from build123d import *

# Parameters (mm, degrees)
SKETCH_1_R          = 3
EXTRUDE_1_DEPTH     = 1
SKETCH_2_R          = 1.5
EXTRUDE_2_DEPTH     = 4
FILLET_1_R          = 0.4
CUT_EXTRUDE_1_DEPTH = 0.7
CHAMFER_1_SIZE      = 0.1
CHAMFER_2_SIZE      = 0.3


with BuildPart() as part:
    # 草图1 → 凸台-拉伸1 (new body)
    with BuildSketch(Plane.XY):
        Circle(SKETCH_1_R)
    extrude(amount=EXTRUDE_1_DEPTH)

    # 草图2 → 凸台-拉伸2 (add)
    with BuildSketch(Plane(origin=(0, 0, 0), x_dir=(-1, 0, 0), z_dir=(0, 0, -1))):
        Circle(SKETCH_2_R)
    extrude(amount=EXTRUDE_2_DEPTH)

    # 圆角1
    fillet_1_edges = [part.edges().sort_by_distance(p)[0] for p in [
        (-3, 0, 0),
        (-3, 0, 1),
    ]]
    fillet(fillet_1_edges, radius=FILLET_1_R)

    # 草图3 → 切除-拉伸1 (cut)
    with BuildSketch(Plane.XY.offset(1)):
        Polygon((0.343622422, -1.10238694), (1.126506305, -0.253607723), (0.782883884, 0.848779216), (-0.343622422, 1.10238694), (-1.126506305, 0.253607723), (-0.782883884, -0.848779216), align=None)
    extrude(amount=-CUT_EXTRUDE_1_DEPTH, mode=Mode.SUBTRACT)

    # 倒角1
    chamfer_1_edges = [part.edges().sort_by_distance(p)[0] for p in [
        (-0.219630731, -0.975583078, 0.3),
        (-0.954695095, -0.297585747, 0.3),
        (-0.735064364, 0.677997331, 0.3),
        (0.219630731, 0.975583078, 0.3),
        (0.954695095, 0.297585747, 0.3),
        (0.735064364, -0.677997331, 0.3),
        (-0.219630731, -0.975583078, 1),
        (0.735064364, -0.677997331, 1),
        (0.954695095, 0.297585747, 1),
        (0.219630731, 0.975583078, 1),
        (-0.735064364, 0.677997331, 1),
        (-0.954695095, -0.297585747, 1),
    ]]
    chamfer(chamfer_1_edges, length=CHAMFER_1_SIZE)

    # 倒角2
    chamfer_2_edges = [part.edges().sort_by_distance(p)[0] for p in [
        (1.5, 0, -4),
    ]]
    chamfer(chamfer_2_edges, length=CHAMFER_2_SIZE)


solid = part.part
Design review of the part built by this model. Coordinates are the model's own, in mm. A direction names the side the tool comes from. Give positions to 0.01 mm unless a question says otherwise; leave off trailing zeros. Order: outer loops, then holes, each group sorted by start corner. A loop starts at its lowest first (then second) coordinate and runs counter-clockwise, first axis right, second up. Notation, with made-up numbers: (30, 33) - (78, 33) arc R16 ccw to (78, 58) - close; hole circle Ø4 at (21, 64.25). An arc over 180 degrees is marked (long way). Use CSV: the item, a comma, the result in double quotes. Start each with the question number.
Q1. Take a section at C-C (z = -0.1). State the section outline as (x, y) points.
Q2. Draft analysis for pull direction Y (two halves, no side actions). For faces 3 (the face through (0, 0, 0.3)), 4 (the face through (0, 0, -4)), 5 (the face through (1.5, 0.07, -1.82)), state which applies: pulls with the +Y half, pulls with the -Y half, needs draft (parallel to the pull), parting line crosses it, or undercut.
Q3. Take a section at B-B (x = 0). State the section outline as (y, z) points, and give its area (3 significant figures).
Q4. For P1, Ø3, axis at y = 2, z = -3, coming from the +X side; P2, Ø3, axis at y = -1.5, z = -3, coming from the +X side; P3, Ø2, axis at x = 1.5, z = 0, coming from the -Y side, all flat-tipped, find the tip position at first contact; note any pin that passes through.
Q5. Take a section at A-A (y = 0). State the section outline as (x, z) points.
Q6. For line 1 (Z direction, x = 0.1, y = 0.7); line 2 (Z direction, x = 0.5, y = -2.4); line 3 (Y direction, x = -0.45, z = -2.15), list the stretches that pass through material, from the lowest coordinate up.
Q7. Machinability: for faces 1 (the face through (1, -1, 1)), 2 (the face through (2, 0, 0)), which of the approach directions +Z, -Z, +X, -X, +Y, -Y give a long, thin tool a straight path to every point of the face, cutting with its end or side? Answer none if there is none.
Calculated:
1,outline,"circle Ø3 at (0, 0)"
2,face 3,"undercut"
2,face 4,"needs draft"
2,face 5,"parting line crosses it"
3,outline,"(-3, 0.4) arc R0.4 ccw to (-2.6, 0) - (-1.5, 0) - (-1.5, -3.7) - (-1.2, -4) - (1.2, -4) - (1.5, -3.7) - (1.5, 0) - (2.6, 0) arc R0.4 ccw to (3, 0.4) - (3, 0.6) arc R0.4 ccw to (2.6, 1) - (1.13, 1) - (1.03, 0.9) - (1.03, 0.4) - (0.92, 0.3) - (-0.92, 0.3) - (-1.03, 0.4) - (-1.03, 0.9) - (-1.13, 1) - (-2.6, 1) arc R0.4 ccw to (-3, 0.6) - close"
3,area,"16.3 mm²"
4,P1,"stops at x = 1.41"
4,P2,"stops at x = 1.5"
4,P3,"stops at y = -2.94"
5,outline,"(-3, 0.4) arc R0.4 ccw to (-2.6, 0) - (-1.5, 0) - (-1.5, -3.7) - (-1.2, -4) - (1.2, -4) - (1.5, -3.7) - (1.5, 0) - (2.6, 0) arc R0.4 ccw to (3, 0.4) - (3, 0.6) arc R0.4 ccw to (2.6, 1) - (1.15, 1) - (1.05, 0.9) - (1.05, 0.4) - (0.94, 0.3) - (-0.94, 0.3) - (-1.05, 0.4) - (-1.05, 0.9) - (-1.15, 1) - (-2.6, 1) arc R0.4 ccw to (-3, 0.6) - close"
6,line 1,"z = -4 to 0.3"
6,line 2,"z = 0 to 1"
6,line 3,"y = -1.43 to 1.43"
7,face 1,"+Z, +X, -X, +Y, -Y"
7,face 2,"-Z"
